Autodesk Inventor part; units mm, degrees
ref_plane "YZ Plane" through (0, 0, 0) normal (1, 0, 0) x (0, 1, 0)
ref_plane "XZ Plane" through (0, 0, 0) normal (0, 1, 0) x (-1, 0, 0)
ref_plane "XY Plane" through (0, 0, 0) normal (0, 0, 1) x (1, 0, 0)
sketch "Sketch1" plane through (0, 0, 0) normal (0, 0, 1) x (1, 0, 0)
  line L0 (0, 0) -> (85.5, 0)
  line L1 (85.5, 0) -> (85.5, -116.825)
  line L2 (85.5, -116.825) -> (0, -116.825)
  line L3 (0, -116.825) -> (0, 0)
  dimension "d0" = 85.5
  dimension "d1" = 116.825
extrude "Extrusion1" add sketch "Sketch1" along normal blind 2
sketch "Sketch2" plane through (0, 0, 0) normal (0, 0, -1) x (-1, 0, 0)
  line L0 (-85.5, 0) -> (0, 0)
  line L1 (0, 0) -> (-42.75, 0)
  line L2 (-42.75, 0) -> (-47.75, 0)
  line L3 (-47.75, 0) -> (-37.75, 0)
  line L4 (-37.75, 0) -> (-37.75, 10)
  line L5 (-37.75, 10) -> (-47.75, 10)
  line L6 (-47.75, 10) -> (-47.75, 0)
  dimension "d4" = 5
  dimension "d5" = 10
  dimension "d6" = 10
extrude "Extrusion2" add sketch "Sketch2" against normal blind 2
sketch "Sketch3" plane through (0, 0, 2) normal (0, 0, 1) x (1, 0, 0)
  line L0 (0, 0) -> (37.75, 0)
  line L1 (37.75, 0) -> (37.75, -13.175)
  line L2 (37.75, -13.175) -> (47.75, -13.175)
  line L3 (47.75, 0) -> (47.75, 10)
  line L4 (47.75, -13.175) -> (47.75, 0)
  line L5 (47.75, 0) -> (48.75, 0)
  line L6 (47.75, 0) -> (85.5, 0)
  line L7 (48.75, 0) -> (48.75, -13.175)
  line L8 (48.75, -13.175) -> (48.75, -14.175)
  line L9 (48.75, -14.175) -> (37.75, -14.175)
  line L10 (37.75, -14.175) -> (36.75, -14.175)
  line L11 (36.75, -14.175) -> (36.75, 0)
  line L12 (37.75, -13.175) -> (37.75, -14.175)
  line L13 (47.75, -13.175) -> (47.75, -14.175)
  dimension "d9" = 13.175
  dimension "d10" = 1
  dimension "d11" = 1
  dimension "d12" = 1
extrude "Extrusion3" cut sketch "Sketch3" against normal blind 3.175 contours L0 L1 L12 L10 L11 | L4 L5 L7 L8 L9 L13
sketch "Sketch4" plane through (0, 0, 2) normal (0, 0, 1) x (1, 0, 0)
  line L0 (37.75, 10) -> (37.75, -14.175)
  line L1 (47.75, -14.175) -> (47.75, 10)
  line L2 (37.75, 0) -> (47.75, 0)
  line L3 (47.75, 0) -> (47.75, -4)
  line L4 (47.75, -4) -> (37.75, -4)
  line L5 (37.75, -4) -> (37.75, 0)
  point P0 (0, 0)
  dimension "d15" = 4
extrude "Extrusion4" add sketch "Sketch4" along normal blind 2
fillet "Fillet1" radius 2 2 edges at (42.75, 0, 4) (42.75, -4, 4)
fillet "Fillet2" radius 2 3 edges at (0, -116.825, 1) (85.5, -116.825, 1) (42.75, -116.825, 2)
fillet "Fillet3" radius 2 2 edges at (37.75, 10, 1) (47.75, 10, 1)
properties part number "BatteryBoxLid"
Here's how the part is built. I have some questions about the finished solid (model axes, mm). Coordinates: 2 decimals unless noted, no trailing zeros. Loops run counter-clockwise (first coordinate to the right, second up) from the corner with the lowest first, then second, coordinate; pieces in that order, holes last. Notation, with made-up numbers: M 18,21.5 L 48,21.5 A11 ccw 48,33.5 Z; hole C -13.75,3 d9. An arc over 180 degrees is marked long. One line per item, written item: value.
1. Thinking about a two-plate mould opening in X: for faces 1 (the flat face through (43, 5, 2)), 2 (the flat face through (47.75, -3, 1)), 3 (the flat face through (37.75, -3, 1)), which applies, +X half, -X half, draft (parallel to the pull), parting line (faces both ways), or undercut?
Geometry says:
face 1: draft
face 2: undercut
face 3: undercut
2. Will these pins go through, and if not, where does the flat tip stop? pin 1 Ø0.8 at (x, z) = (48.5, 1) entering from +Y; pin 2 Ø3 at (x, y) = (36.5, -52) entering from +Z.
Geometry says:
pin 1: stops at y = 0
pin 2: stops at z = 2
3. Please list where these lines run through material, in increasing order: probe 1 along Z at (x, y) = (81, -92.5); probe 2 along Y at (x, z) = (24.5, 1.8); probe 3 along Y at (x, z) = (28.5, 0.75).
Geometry says:
probe 1: z = 0 to 2
probe 2: y = -115.7 to 0
probe 3: y = -116.68 to 0
4. Imagine slicing it at A-A (y = -6.5). List the corners of the cut face in (x, z) for me.
Geometry says:
outline: M 0,0 L 36.75,0 L 36.75,2 L 0,2 Z; M 37.75,0 L 47.75,0 L 47.75,2 L 37.75,2 Z; M 48.75,0 L 85.5,0 L 85.5,2 L 48.75,2 Z
